CAD build for the part. Positions are in the model's coordinates, mm. A direction names the side the tool comes from. Give positions to 0.01 mm unless a question says otherwise; leave off trailing zeros. Order: outer loops, then holes, each group sorted by start corner. A loop starts at its lowest first (then second) coordinate and runs counter-clockwise, first axis right, second up. Notation, with made-up numbers: (74, 85.5) -> (123, 85.5) arc R27 ccw to (123, 120.5) -> close; hole circle Ø11 at (84.25, 19). An arc over 180 degrees is marked (long way). Use one line per item in the form item = value. Start each with the question number.
1) Cut at A-A, the plane z = 12.7. Give the cut face in (x, y) (3 decimals), and give its area (3 significant figures).
2) Cut at D-D, the plane z = -17.5. Give the cut face in (x, y).
3) Cut at B-B, the plane y = -12.7. Give the cut face in (x, z), and give its area (3 significant figures).
4) Tool access for faces 1 (the face through (0, 22.86, 0)), 2 (the face through (-11.412, -12.591, -10.213)): list every direction of +Z, -Z, +X, -X, +Y, -Y with a clear straight run to the whole face (end or side of a thin tool).
5) Cut at C-C, the plane x = -7.75. Give the cut face in (y, z), and give its area (3 significant figures).
6) Mould opens along Z. For faces 3 (the face through (-10.4, 2, 25.4)), 4 (the face through (-10.4, 2, -25.4)), 5 (the face through (1.5, 24.1, -9.9)), 6 (the face through (10.16, 0, 0)) say: pulls with the +Z half, pulls with the -Z half, needs draft (parallel to the pull), parting line crosses it, or undercut.
7) Probe line 1 (Z direction, x = 0, y = -24.05) (3 decimals); line 2 (Y direction, x = -11.65, z = -12.7); line 3 (Y direction, x = -3.5, z = 10). List the from-to ranges inside material, lowest first.
from build123d import *

# Parameters (mm, degrees)
SKETCH1_W           = 25.4
SKETCH1_H           = 50.8
SKETCH1_W_2         = 20.32
SKETCH1_H_2         = 45.72
EXTRUDE_THIN1_DEPTH = 25.4
SKETCH2_R           = 3.175
CUT_EXTRUDE1_DEPTH  = 51.8
SKETCH3_R           = 2.4892
CUT_EXTRUDE2_DEPTH  = 26.4


with BuildPart() as part:
    # Sketch1 → Extrude-Thin1 (new body, symmetric)
    with BuildSketch(Plane.XY):
        Rectangle(SKETCH1_W, SKETCH1_H)
        Rectangle(SKETCH1_W_2, SKETCH1_H_2, mode=Mode.SUBTRACT)
    extrude(amount=EXTRUDE_THIN1_DEPTH, both=True)

    # Sketch2 → Cut-Extrude1 (cut, through all)
    with BuildSketch(Plane(origin=(0, 25.4, 0), x_dir=(1, 0, 0), z_dir=(0, 1, 0))):
        with Locations((0, 12.7)):
            Circle(SKETCH2_R)
        with Locations((0, -12.7)):
            Circle(SKETCH2_R)
    extrude(amount=-CUT_EXTRUDE1_DEPTH, mode=Mode.SUBTRACT)

    # Sketch3 → Cut-Extrude2 (cut, through all)
    with BuildSketch(Plane(origin=(12.7, 0, 0), x_dir=(0, 0, -1), z_dir=(1, 0, 0))):
        with Locations((12.7, 12.7)):
            Circle(SKETCH3_R)
        with Locations((12.7, -12.7)):
            Circle(SKETCH3_R)
    extrude(amount=-CUT_EXTRUDE2_DEPTH, mode=Mode.SUBTRACT)


solid = part.part
Result:
q1.outline = (-12.7, -25.4) -> (-3.175, -25.4) -> (-3.175, -22.86) -> (-10.16, -22.86) -> (-10.16, 22.86) -> (-3.175, 22.86) -> (-3.175, 25.4) -> (-12.7, 25.4) -> close; (3.175, -25.4) -> (12.7, -25.4) -> (12.7, 25.4) -> (3.175, 25.4) -> (3.175, 22.86) -> (10.16, 22.86) -> (10.16, -22.86) -> (3.175, -22.86) -> close
q1.area = 329 mm²
q2.outline = (-12.7, -25.4) -> (12.7, -25.4) -> (12.7, 25.4) -> (-12.7, 25.4) -> close; hole (-10.16, -22.86) -> (10.16, -22.86) -> (10.16, 22.86) -> (-10.16, 22.86) -> close
q3.outline = (-12.7, -25.4) -> (-10.16, -25.4) -> (-10.16, -15.19) -> (-12.7, -15.19) -> close; (-12.7, -10.21) -> (-10.16, -10.21) -> (-10.16, 25.4) -> (-12.7, 25.4) -> close; (10.16, -25.4) -> (12.7, -25.4) -> (12.7, -15.19) -> (10.16, -15.19) -> close; (10.16, -10.21) -> (12.7, -10.21) -> (12.7, 25.4) -> (10.16, 25.4) -> close
q3.area = 233 mm²
q4.face_1 = +Z, -Z
q4.face_2 = +X, -X
q5.outline = (-25.4, -25.4) -> (-22.86, -25.4) -> (-22.86, 25.4) -> (-25.4, 25.4) -> close; (22.86, -25.4) -> (25.4, -25.4) -> (25.4, 25.4) -> (22.86, 25.4) -> close
q5.area = 258 mm²
q6.face_3 = pulls with the +Z half
q6.face_4 = pulls with the -Z half
q6.face_5 = undercut
q6.face_6 = needs draft
q7.line_1 = -25.4 to -15.875, -9.525 to 9.525, 15.875 to 25.4
q7.line_2 = -25.4 to -15.19, -10.21 to 10.21, 15.19 to 25.4
q7.line_3 = -25.4 to -22.86, 22.86 to 25.4
